Can you work these out from the model? Positions are in its coordinate system, mm. Coordinates: 2 decimals unless noted, no trailing zeros. Loops run counter-clockwise (first coordinate to the right, second up) from the corner with the lowest first, then second, coordinate; pieces in that order, holes last. Notation, with made-up numbers: (29, 62.5) -> (46, 62.5) arc R20 ccw to (46, 84.5) -> close; hole circle Ø2 at (26.5, 76.5). An arc over 180 degrees is marked (long way). Put each result on its own line as item: value. Start each with the question number.
Item 1: Please list where these lines run through material, in increasing order: L1, parallel to X at y = 3, z = -116 (3 decimals); L2, parallel to X at y = 38, z = -171; L3, parallel to Y at x = -3, z = -403. Write a range as from..to.
Item 2: Will these pins go through, and if not, where does the flat tip stop? P1, Ø1.1, axis at x = -1.5, z = -150, coming from the +Y side; P2, Ø5.5, axis at x = -8.5, z = -341, coming from the -Y side; P3, Ø1, axis at x = -10, z = -93, coming from the -Y side; P4, Ø8, axis at x = -12.5, z = -380, coming from the -Y side.
Item 3: If we section it at B-B on y = 24: Please give me the cut outline in (x, z) (3 decimals).
Item 4: If we section it at A-A on z = -404: Please give me the cut outline in (x, y) (3 decimals), plus the area to 3 significant figures.
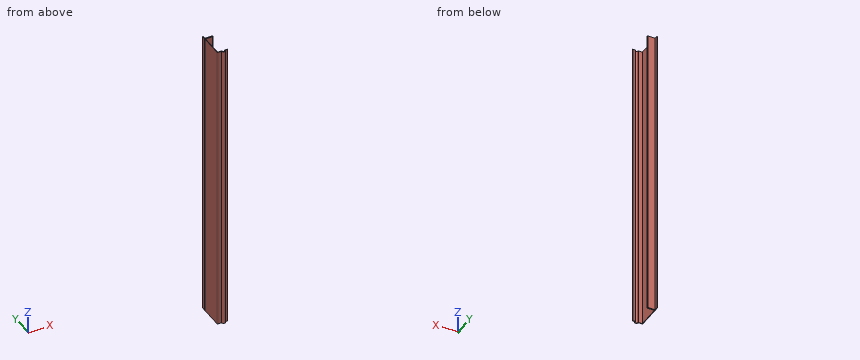
```python
from build123d import *

# Parameters (mm, degrees)
EXTRUDE_THIN1_DEPTH = 464.34375
FILLET1_R           = 0.889


with BuildPart() as part:
    # Sketch1 → Extrude-Thin1 (new body)
    with BuildSketch(Plane.XY):
        with BuildLine():
            Line((-15.875, 43.65625), (-15.875, 37.35705))
            Line((-15.875, 37.35705), (-4.1148, 37.35705))
            ThreePointArc((-4.1148, 37.35705), (-4.064, 37.30625), (-4.1148, 37.25545))
            Line((-4.1148, 37.25545), (-15.875, 37.25545))
            Line((-15.875, 37.25545), (-15.875, 0))
            Line((-15.875, 0), (-9.128125, 0))
            ThreePointArc((-9.128125, 0), (-6.35, -2.778125), (-3.571875, 0))
            Line((-3.571875, 0), (0, 0))
            Line((0, 0), (0, 0.889))
            Line((0, 0.889), (-4.683125, 0.889))
            ThreePointArc((-4.683125, 0.889), (-6.35, -1.889125), (-8.016875, 0.889))
            Line((-8.016875, 0.889), (-14.986, 0.889))
            Line((-14.986, 0.889), (-14.986, 36.36645))
            Line((-14.986, 36.36645), (-4.1148, 36.36645))
            ThreePointArc((-4.1148, 36.36645), (-3.175, 37.30625), (-4.1148, 38.24605))
            Line((-4.1148, 38.24605), (-14.986, 38.24605))
            Line((-14.986, 38.24605), (-14.986, 43.65625))
            Line((-14.986, 43.65625), (-15.875, 43.65625))
        make_face()
    extrude(amount=-EXTRUDE_THIN1_DEPTH)

    # Fillet1
    fillet1_edges = [part.edges().sort_by_distance(p)[0] for p in [
        (-15.875, 0, -232.171875),
        (-15.875, 37.25545, -232.171875),
        (-15.875, 37.35705, -232.171875),
        (-8.016875, 0.889, -232.171875),
        (-4.683125, 0.889, -232.171875),
    ]]
    fillet(fillet1_edges, radius=FILLET1_R)


solid = part.part
```
Solutions:
1. L1: -15.875..-14.986
1. L2: -15.84..-3.48
1. L3: 0..0.89
2. P1: y = 0.89
2. P2: y = -2.78
2. P3: y = 0
2. P4: y = -1.76
3. outline: (-15.875, -464.344) -> (-14.986, -464.344) -> (-14.986, 0) -> (-15.875, 0) -> close
4. outline: (-15.875, 0.889) arc R0.889 ccw to (-14.986, 0) -> (-9.128, 0) arc R2.778 ccw to (-3.572, 0) -> (0, 0) -> (0, 0.889) -> (-3.572, 0.889) arc R0.889 ccw to (-4.461, 0) arc R1.889 cw to (-8.239, 0) arc R0.889 ccw to (-9.128, 0.889) -> (-14.986, 0.889) -> (-14.986, 36.366) -> (-4.115, 36.366) arc R0.94 ccw to (-4.115, 38.246) -> (-14.986, 38.246) -> (-14.986, 43.656) -> (-15.875, 43.656) -> (-15.875, 38.246) arc R0.889 ccw to (-14.986, 37.357) -> (-4.115, 37.357) arc R0.051 cw to (-4.115, 37.255) -> (-14.986, 37.255) arc R0.889 ccw to (-15.875, 36.366) -> close
4. area: 75.1 mm^2
